The listing builds one solid part. Answer for the finished solid, in the listing's coordinates (mm). Face numbers are marked on the shaded views. A direction names the side the tool comes from. Round coordinates to 2 decimals unless told otherwise and drop trailing zeros. Write each loop counter-clockwise with the first axis right and the second up, starting at its lowest first coordinate (ties: lowest second). Pieces come first, ordered by that corner, then holes. Notation, with made-up numbers: (-23.5, -40) - (32.5, -40) arc R22 ccw to (32.5, -5) - close; hole circle Ø1 at (61.25, 49.25). An arc over 180 degrees is marked (long way). Return JSON: item names as keys, results as strings. Group by question number.
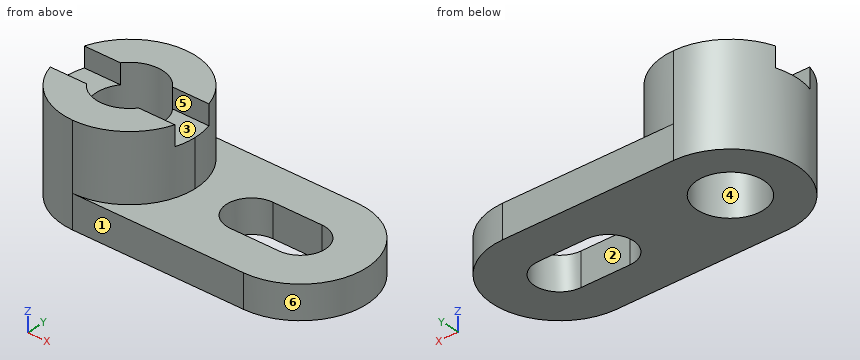
from build123d import *

# Parameters (mm, degrees)
F1_DEPTH = 10
F3_DEPTH = 20
F4_R     = 10
F5_DEPTH = 50
F7_DEPTH = 6
F9_DEPTH = 25


with BuildPart() as f1:
    # F0 (on Top) → F1 (new body)
    with BuildSketch(Plane.XY):
        with BuildLine():
            Line((52.3521453142, 20), (0, 20))
            ThreePointArc((0, 20), (-20, 0), (0, -20))
            Line((0, -20), (52.3521453142, -20))
            ThreePointArc((52.3521453142, -20), (72.3521453142, 0), (52.3521453142, 20))
        make_face()
    extrude(amount=F1_DEPTH)

    # F2 (on face) → F3 (join)
    with BuildSketch(Plane.XY.offset(10)):
        with BuildLine():
            ThreePointArc((0, -20), (14.1421356237, -14.1421356237), (20, 0))
            ThreePointArc((20, 0), (14.1421356237, 14.1421356237), (0, 20))
            ThreePointArc((0, 20), (-20, 0), (0, -20))
        make_face()
    extrude(amount=F3_DEPTH)

    # F4 (on face) → F5 (cut)
    with BuildSketch(Plane.XY.offset(30)):
        Circle(F4_R)
    extrude(amount=-F5_DEPTH, mode=Mode.SUBTRACT)

    # F6 (on face) → F7 (cut)
    with BuildSketch(Plane.XY.offset(30)):
        with BuildLine():
            Line((24.870807305, 6.0082398243), (19.0761907679, 6.0082398243))
            ThreePointArc((19.0761907679, 6.0082398243), (19.7676985934, 3.0394230244), (20, 0))
            ThreePointArc((20, 0), (19.7690094284, -3.0308853852), (19.0813733782, -5.9917601757))
            Line((19.0813733782, -5.9917601757), (24.870807305, -5.9917601757))
            Line((24.870807305, -5.9917601757), (24.870807305, 6.0082398243))
        make_face()
        with BuildLine():
            Line((-7.9938134963, 6.0082398243), (-19.0761907679, 6.0082398243))
            ThreePointArc((-19.0761907679, 6.0082398243), (-19.9999981348, 0.008637683), (-19.0813733782, -5.9917601757))
            Line((-19.0813733782, -5.9917601757), (-8.006173243, -5.9917601757))
            ThreePointArc((-8.006173243, -5.9917601757), (-9.9999946957, 0.0102997835), (-7.9938134963, 6.0082398243))
        make_face()
        with BuildLine():
            Line((7.9938134963, 6.0082398243), (-7.9938134963, 6.0082398243))
            ThreePointArc((-7.9938134963, 6.0082398243), (-9.9999946957, 0.0102997835), (-8.006173243, -5.9917601757))
            Line((-8.006173243, -5.9917601757), (8.006173243, -5.9917601757))
            ThreePointArc((8.006173243, -5.9917601757), (9.4884596334, -3.1573935113), (10, 0))
            ThreePointArc((10, 0), (9.4852025535, 3.1671647445), (7.9938134963, 6.0082398243))
        make_face()
        with BuildLine():
            ThreePointArc((20, 0), (19.7676985934, 3.0394230244), (19.0761907679, 6.0082398243))
            Line((19.0761907679, 6.0082398243), (7.9938134963, 6.0082398243))
            ThreePointArc((7.9938134963, 6.0082398243), (9.4852025535, 3.1671647445), (10, 0))
            ThreePointArc((10, 0), (9.4884596334, -3.1573935113), (8.006173243, -5.9917601757))
            Line((8.006173243, -5.9917601757), (19.0813733782, -5.9917601757))
            ThreePointArc((19.0813733782, -5.9917601757), (19.7690094284, -3.0308853852), (20, 0))
        make_face()
    extrude(amount=-F7_DEPTH, mode=Mode.SUBTRACT)

    # F8 (on face) → F9 (cut)
    with BuildSketch(Plane.XY.offset(10)):
        with BuildLine():
            Line((52.3521453142, 7.5), (37.3521453142, 7.5))
            ThreePointArc((37.3521453142, 7.5), (29.8521453142, 0), (37.3521453142, -7.5))
            Line((37.3521453142, -7.5), (52.3521453142, -7.5))
            ThreePointArc((52.3521453142, -7.5), (59.8521453142, 0), (52.3521453142, 7.5))
        make_face()
    extrude(amount=-F9_DEPTH, mode=Mode.SUBTRACT)


solid = f1.part
(1) For the marked faces 1, 2 and 3, determine the directions among +Z, -Z, +X, -X, +Y, -Y from which every point of the face is accessible in a straight line to the end or side of a thin tool.
(2) Determine the mould class of the marked faces 4, 5 and 6 for opening direction X: +X half, -X half, draft (parallel to the pull), parting line (faces both ways), or undercut.
(3) Flat-ended cylindrical pins translate along their axes: pin 1 (4 mm diameter, centred on y = -11.5, z = 5, fed in from -X); pin 2 (1 mm diameter, centred on x = 58.5, y = -9, fed in from -Z); pin 3 (6 mm diameter, centred on x = 16, y = -2, fed in from +Z); pin 4 (2 mm diameter, centred on y = 3, z = 17.5, fed in from +X). Find the tip coordinate at first contact, or state that the pin passes through.
(4) Find section B-B (x = 31). Write down the section's boundary in (y, z).
(5) Find section D-D (y = -17). Write down the section's boundary in (x, z), plus the area to 3 significant figures.
(6) Find section A-A (z = 9). Write down the section's boundary in (x, y).
(7) Consider line 1 (Y direction, x = 51.5, z = 9); line 2 (Z direction, x = 23, y = 0); line 3 (X direction, y = 0, z = 11.75). Determine where each line is inside the solid, lowest interval first.
(8) Find section C-C (y = 17.5). Write down the section's boundary in (x, z), plus the area to 3 significant figures.
Check sheet entries:
{
 "1": {"face 1": "+Z, -Z, +X, -X, -Y", "face 2": "+Z, -Z", "face 3": "+Z, +X, -X"},
 "2": {"face 4": "undercut", "face 5": "draft", "face 6": "+X half"},
 "3": {"pin 1": "stops at x = -17.6", "pin 2": "stops at z = 0", "pin 3": "stops at z = 24", "pin 4": "stops at x = 19.9"},
 "4": {"outline": "(-20, 0) - (-3.99, 0) - (-3.99, 10) - (-20, 10) - close; (3.99, 0) - (20, 0) - (20, 10) - (3.99, 10) - close"},
 "5": {"outline": "(-10.54, 0) - (62.89, 0) - (62.89, 10) - (10.54, 10) - (10.54, 30) - (-10.54, 30) - close", "area": "1,160 mm^2"},
 "6": {"outline": "(0, -20) - (52.35, -20) arc R20 ccw to (52.35, 20) - (0, 20) arc R20 ccw to start; hole circle Ø20 at (0, 0); hole (37.35, -7.5) - (52.35, -7.5) arc R7.5 ccw to (52.35, 7.5) - (37.35, 7.5) arc R7.5 ccw to start"},
 "7": {"line 1": "y = -20 to -7.5, 7.5 to 20", "line 2": "z = 0 to 10", "line 3": "x = -20 to -10, 10 to 20"},
 "8": {"outline": "(-9.68, 0) - (62.03, 0) - (62.03, 10) - (9.68, 10) - (9.68, 30) - (-9.68, 30) - close", "area": "1,100 mm^2"}
}
